Input: part model. Units: mm. Frame: model coordinates. Face numbers are marked on the shaded views. A direction names the side the tool comes from. Coordinates: 2 decimals unless noted, no trailing zeros. Loops run counter-clockwise (first coordinate to the right, second up) from the corner with the lowest first, then second, coordinate; pieces in that order, holes last.
(1) Section A-A, the plane z = 2.5. Return loops of the section in (x, y), then the cut area to 3 significant figures.
(2) Contact query for flat-ended pins moving along their axis: P1, Ø0.6, axis at x = 31, z = 1, coming from the -Y side; P2, Ø1.6, axis at x = 27, z = 4.5, coming from the -Y side; P3, Ø2, axis at y = 6, z = 3.5, coming from the +X side; P4, Ø12, axis at x = 22.5, y = -12, coming from the -Z side. Output: stop coordinate, or through.
(3) Set-up query: the marked faces 1, 2 and 3. Return all of +Z, -Z, +X, -X, +Y, -Y with unobstructed straight access to the full face (end or side cutting, diameter ignored); none if empty.
(4) Section C-C, the plane y = -3.75. Return loops of the section in (x, z).
(5) Section B-B, the plane y = -9. Return loops of the section in (x, z).
(6) Line query: L1, parallel to Y at x = 9.5, z = 2.9; L2, parallel to Y at x = 31, z = 4.05; L3, parallel to X at y = -2, z = 3. Output: solid intervals per line, ascending.
(7) Section D-D, the plane x = 16. Return loops of the section in (y, z).
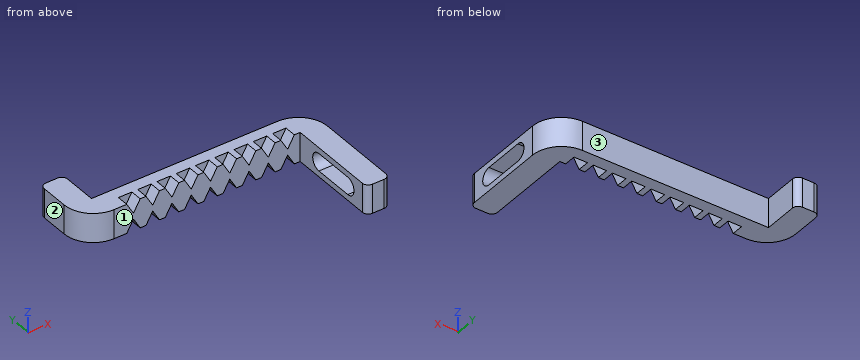
```python
from build123d import *

# Parameters (mm, degrees)
BOSS_EXTRUDE1_DEPTH = 5
CUT_EXTRUDE1_DEPTH  = 41.620192023
FILLET2_R           = 5
FILLET3_R           = 1
CUT_EXTRUDE2_DEPTH  = 2


with BuildPart() as part:
    # Sketch1 → Boss-Extrude1 (new body)
    with BuildSketch(Plane.XY):
        Polygon((0, 0), (33, 0), (33, -16), (37, -16), (37, 4), (0, 4), (0, 10.75), (-4, 10.75), (-4, 0), align=None)
    extrude(amount=BOSS_EXTRUDE1_DEPTH)

    # Sketch3 → Cut-Extrude1 (cut, through all)
    with BuildSketch(Plane.ZY.offset(-33)):
        with BuildLine():
            Line((4, -4.524146601), (4, -11.475853399))
            ThreePointArc((4, -11.475853399), (2.5, -12.975853399), (1, -11.475853399))
            Line((1, -11.475853399), (1, -4.524146601))
            ThreePointArc((1, -4.524146601), (2.5, -3.024146601), (4, -4.524146601))
        make_face()
    extrude(amount=-CUT_EXTRUDE1_DEPTH, mode=Mode.SUBTRACT)

    # Fillet2
    fillet2_edges = [part.edges().sort_by_distance(p)[0] for p in [
        (-4, 0, 2.5),
        (37, 4, 2.5),
    ]]
    fillet(fillet2_edges, radius=FILLET2_R)

    # Fillet3
    fillet3_edges = [part.edges().sort_by_distance(p)[0] for p in [
        (-4, 10.75, 2.5),
        (0, 10.75, 2.5),
        (37, -16, 2.5),
        (33, -16, 2.5),
    ]]
    fillet(fillet3_edges, radius=FILLET3_R)

    # Sketch4 → Cut-Extrude2 (cut)
    with BuildSketch(Plane(origin=(0, 0, 0), x_dir=(-1, 0, 0), z_dir=(0, -1, 0))):
        Polygon((-30.845299462, -3), (-32, -5), (-29.690598923, -5), align=None)
        Polygon((-30.845299462, -2), (-29.690598923, 0), (-32, 0), align=None)
        Polygon((-27.535299462, -3), (-28.69, -5), (-26.380598923, -5), align=None)
        Polygon((-27.535299462, -2), (-26.380598923, 0), (-28.69, 0), align=None)
        Polygon((-24.225299462, -3), (-25.38, -5), (-23.070598923, -5), align=None)
        Polygon((-24.225299462, -2), (-23.070598923, 0), (-25.38, 0), align=None)
        Polygon((-20.915299462, -3), (-22.07, -5), (-19.760598923, -5), align=None)
        Polygon((-20.915299462, -2), (-19.760598923, 0), (-22.07, 0), align=None)
        Polygon((-17.605299462, -3), (-18.76, -5), (-16.450598923, -5), align=None)
        Polygon((-17.605299462, -2), (-16.450598923, 0), (-18.76, 0), align=None)
        Polygon((-14.295299462, -3), (-15.45, -5), (-13.140598923, -5), align=None)
        Polygon((-14.295299462, -2), (-13.140598923, 0), (-15.45, 0), align=None)
        Polygon((-10.985299462, -3), (-12.14, -5), (-9.830598923, -5), align=None)
        Polygon((-10.985299462, -2), (-9.830598923, 0), (-12.14, 0), align=None)
        Polygon((-7.675299462, -3), (-8.83, -5), (-6.520598923, -5), align=None)
        Polygon((-7.675299462, -2), (-6.520598923, 0), (-8.83, 0), align=None)
        Polygon((-4.365299462, -3), (-5.52, -5), (-3.210598923, -5), align=None)
        Polygon((-4.365299462, -2), (-3.210598923, 0), (-5.52, 0), align=None)
    extrude(amount=-CUT_EXTRUDE2_DEPTH, mode=Mode.SUBTRACT)


solid = part.part
```
Report:
1. outline: (-4, 5) arc R5 ccw to (1, 0) - (33, 0) - (33, -3.02) - (37, -3.02) - (37, -1) arc R5 ccw to (32, 4) - (0, 4) - (0, 9.75) arc R1 ccw to (-1, 10.75) - (-3, 10.75) arc R1 ccw to (-4, 9.75) - close; (33, -15) arc R1 ccw to (34, -16) - (36, -16) arc R1 ccw to (37, -15) - (37, -12.98) - (33, -12.98) - close
1. area: 204 mm2
2. P1: stops at y = 2
2. P2: stops at y = 0
2. P3: stops at x = 0
2. P4: passes through
3. face 1: +Z, -Z, -X, -Y
3. face 2: +Z, -Z, -X, +Y, -Y
3. face 3: +Z, -Z, +X, +Y
4. outline: (33, 0) - (37, 0) - (37, 1.22) - (33, 1.22) - close; (33, 3.78) - (37, 3.78) - (37, 5) - (33, 5) - close
5. outline: (33, 0) - (37, 0) - (37, 1) - (33, 1) - close; (33, 4) - (37, 4) - (37, 5) - (33, 5) - close
6. L1: y = 0 to 4
6. L2: y = 2 to 4
6. L3: x = 33 to 37
7. outline: (0, 0) - (4, 0) - (4, 5) - (0, 5) - close
